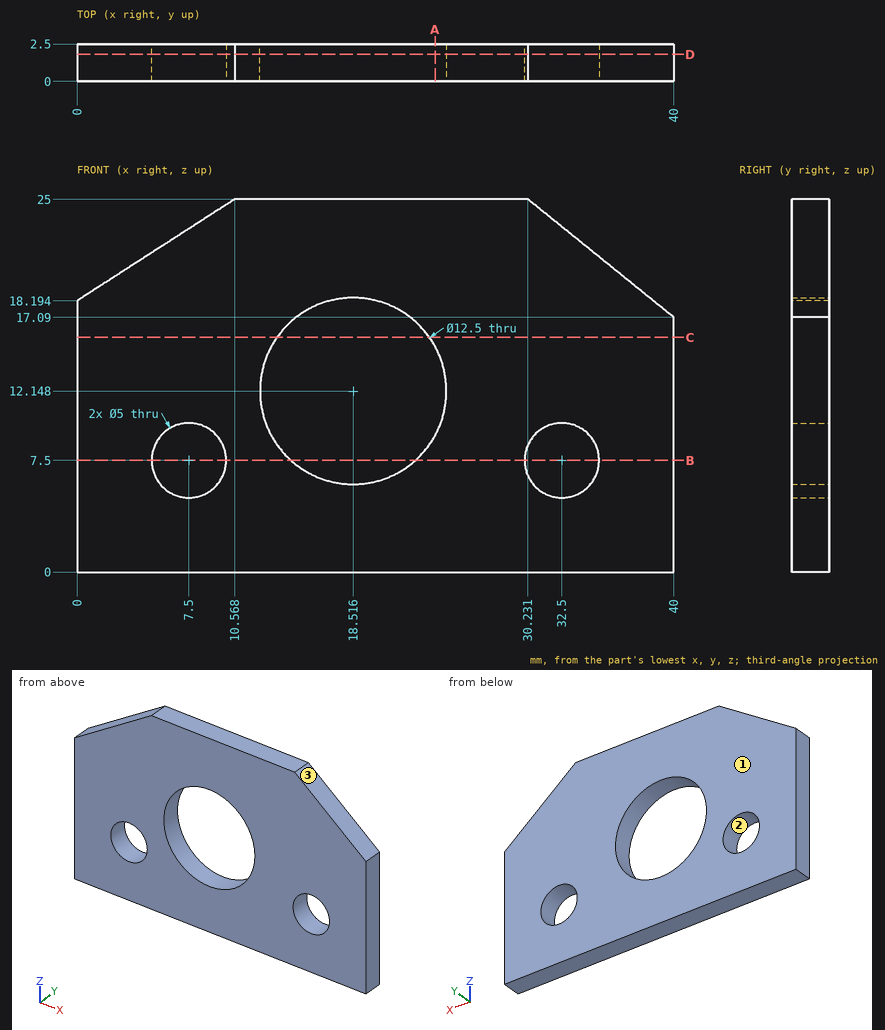
Part print with two shaded views. Sizes in mm from the minimum x, y, z corner. Coordinates: 2 decimals unless noted, no trailing zeros. Loops run counter-clockwise (first coordinate to the right, second up) from the corner with the lowest first, then second, coordinate; pieces in that order, holes last. Notation, with made-up numbers: M 49,81 L 90,81 A19 ccw 90,90 Z; hole C -34,6.25 d7. An arc over 180 degrees is marked long. Use CSV: the item, a comma, the result in double quotes. Start each with the question number.
1. Band-saw the part on C-C, the plane z = 15.75. List the corners of the cut face in (x, y).
2. Band-saw the part on A-A, the plane x = 24. List the corners of the cut face in (y, z).
3. Band-saw the part on D-D, the plane y = 1.8. Give the number of separate pieces and of enclosed holes in the cut face.
4. Flat gauge pin, fed straight in: pin 1 (4.5 mm diameter, centred on x = 7.5, z = 7.5, fed in from -Y). Where does the tip first touch, or does it go through?
5. Probe probe 1 along X at (y, z) = (0.9, 8.5); probe 2 along X at (y, z) = (0.85, 9.5) (1 decimal); probe 3 along Z at (x, y) = (7.5, 1.95) (1 decimal). List the from-to ranges inside material, lowest first. Write a range as [from, to].
6. Two-plate mould, pull along X, no slides. Class the marked faces 1, 2 and 3: pulls with the +X half, pulls with the -X half, needs draft (parallel to the pull), parting line crosses it, or undercut.
7. Band-saw the part on B-B, the plane z = 7.5. List the corners of the cut face in (x, y) (1 decimal).
Entries:
1,outline,"M 0,0 L 13.41,0 L 13.41,2.5 L 0,2.5 Z; M 23.62,0 L 40,0 L 40,2.5 L 23.62,2.5 Z"
2,outline,"M 0,0 L 2.5,0 L 2.5,9.15 L 0,9.15 Z; M 0,15.15 L 2.5,15.15 L 2.5,25 L 0,25 Z"
3,separate pieces,"1"
3,enclosed holes,"3"
4,pin 1,"passes through"
5,probe 1,"x = [0, 5.21], [9.79, 13.44], [23.59, 30.21], [34.79, 40]"
5,probe 2,"x = [0, 6], [9, 12.9], [24.2, 31], [34, 40]"
5,probe 3,"z = [0, 5], [10, 23]"
6,face 1,"needs draft"
6,face 2,"undercut"
6,face 3,"pulls with the +X half"
7,outline,"M 0,0 L 5,0 L 5,2.5 L 0,2.5 Z; M 10,0 L 14.3,0 L 14.3,2.5 L 10,2.5 Z; M 22.7,0 L 30,0 L 30,2.5 L 22.7,2.5 Z; M 35,0 L 40,0 L 40,2.5 L 35,2.5 Z"
